Geometry check sheet. Reference: the model listing, model coordinates, mm. Give positions to 0.01 mm unless a question says otherwise; leave off trailing zeros. Loops run counter-clockwise (first coordinate to the right, second up) from the corner with the lowest first, then second, coordinate; pieces in that order, holes last. Notation, with made-up numbers: (30.5, -29) - (62.5, -29) arc R12 ccw to (62.5, -13) - close; hole circle Ø3 at (-8, 53). An arc over 180 degrees is marked (long way). One line per question, with ' | ' between items. Start each with the question number.
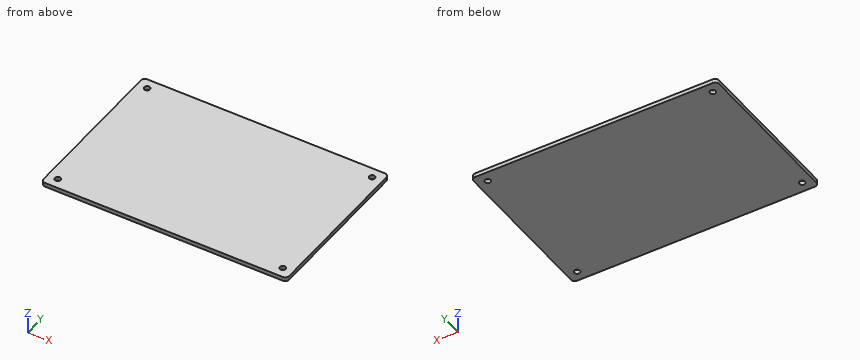
from build123d import *

# Parameters (mm, degrees)
ESQUISSE1_W             = 120
ESQUISSE1_H             = 80
BOSS_EXTRU_1_DEPTH      = 2
CONG_4_R                = 2
CONG_5_R                = 2
ESQUISSE2_R             = 1.407340655
ENL_V_MAT_EXTRU_1_DEPTH = 3


with BuildPart() as part:
    # Esquisse1 → Boss.-Extru.1 (new body)
    with BuildSketch(Plane.XY):
        with Locations((60, 40)):
            Rectangle(ESQUISSE1_W, ESQUISSE1_H)
    extrude(amount=BOSS_EXTRU_1_DEPTH)

    # Congé4
    cong_4_edges = [part.edges().sort_by_distance(p)[0] for p in [
        (0, 0, 1),
    ]]
    fillet(cong_4_edges, radius=CONG_4_R)

    # Congé5
    cong_5_edges = [part.edges().sort_by_distance(p)[0] for p in [
        (0, 80, 1),
        (120, 80, 1),
        (120, 0, 1),
    ]]
    fillet(cong_5_edges, radius=CONG_5_R)

    # Esquisse2 → Enlèv. mat.-Extru.1 (cut, through all)
    with BuildSketch(Plane.XY):
        with Locations((5, 75)):
            Circle(ESQUISSE2_R)
        with Locations((5, 5)):
            Circle(ESQUISSE2_R)
        with Locations((115, 5)):
            Circle(ESQUISSE2_R)
        with Locations((115, 75)):
            Circle(ESQUISSE2_R)
    extrude(amount=ENL_V_MAT_EXTRU_1_DEPTH, mode=Mode.SUBTRACT)


solid = part.part
(1) Section check A-A, the plane y = 75. Record the boundary of the cut face in (x, z), and give its area (3 significant figures).
(2) Material ranges on line 1 (Y direction, x = 115, z = 1.35); line 2 (X direction, y = 5, z = 1.3); line 3 (X direction, y = 75.5, z = 0.15), recorded low to high.
(3) Section check B-B, the plane x = 5. Record the boundary of the cut face in (y, z).
Numbers:
1) outline: (0, 0) - (3.59, 0) - (3.59, 2) - (0, 2) - close; (6.41, 0) - (113.59, 0) - (113.59, 2) - (6.41, 2) - close; (116.41, 0) - (120, 0) - (120, 2) - (116.41, 2) - close | area: 229 mm^2
2) line 1: 0 to 3.59, 6.41 to 73.59, 76.41 to 80 | line 2: 0 to 3.59, 6.41 to 113.59, 116.41 to 120 | line 3: 0 to 3.68, 6.32 to 113.68, 116.32 to 120
3) outline: (0, 0) - (3.59, 0) - (3.59, 2) - (0, 2) - close; (6.41, 0) - (73.59, 0) - (73.59, 2) - (6.41, 2) - close; (76.41, 0) - (80, 0) - (80, 2) - (76.41, 2) - close
